```python
from build123d import *

# Parameters (mm, degrees)
SKETCH1_R           = 2
SKETCH1_R_2         = 1.5
BOSS_EXTRUDE1_DEPTH = 1.5
SCALE1_SCALE        = 1.5
FILLET1_R           = 0.75


with BuildPart() as part:
    # Sketch1 → Boss-Extrude1 (new, symmetric)
    with BuildSketch(Plane(origin=(0, 0, 0), x_dir=(1, 0, 0), z_dir=(0, 1, 0))):
        with BuildLine():
            ThreePointArc((-18.5, 4), (-22.5, 0), (-18.5, -4))
            Line((-18.5, -4), (-12.5, -4))
            ThreePointArc((-12.5, -4), (-10.036924503, -2.516685226), (-7.208497378, -2))
            Line((-7.208497378, -2), (8.627016654, -2))
            ThreePointArc((8.627016654, -2), (10.627016654, -2.254033308), (12.5, -3))
            Line((12.5, -3), (18.5, -3))
            ThreePointArc((18.5, -3), (21.5, 0), (18.5, 3))
            Line((18.5, 3), (12.5, 3))
            ThreePointArc((12.5, 3), (10.627016654, 2.254033308), (8.627016654, 2))
            Line((8.627016654, 2), (-7.208497378, 2))
            ThreePointArc((-7.208497378, 2), (-10.036924503, 2.516685226), (-12.5, 4))
            Line((-12.5, 4), (-18.5, 4))
        make_face()
        with Locations(Location((-18.5, 0, 0), (0, 0, 270))):
            Circle(SKETCH1_R, mode=Mode.SUBTRACT)
        with Locations(Location((18.5, 0, 0), (0, 0, 270))):
            Circle(SKETCH1_R_2, mode=Mode.SUBTRACT)
    extrude(amount=BOSS_EXTRUDE1_DEPTH, both=True)


with BuildPart() as part_1:
    # Scale1: scaled about (-1.682409561, 0, 0)
    add(part.part.scale(SCALE1_SCALE).moved(Location((0.841204781, 0, 0))))

    # Fillet1
    fillet1_edges = [part_1.edges().sort_by_distance(p)[0] for p in [
        (33.09120478, 2.25, 0),
        (24.091204781, 2.25, -4.5),
        (16.781729761, -2.25, 3.381049961),
        (1.905094237, -2.25, 3),
        (-14.214181973, -2.25, 3.77502784),
        (-22.408795219, -2.25, 6),
        (-32.908795219, -2.25, 0),
        (-22.408795219, -2.25, -6),
        (-14.214181973, -2.25, -3.77502784),
        (1.905094237, -2.25, -3),
        (16.781729761, -2.25, -3.381049961),
        (24.091204781, -2.25, -4.5),
        (16.781729761, 2.25, -3.381049961),
        (33.09120478, -2.25, 0),
        (24.091204781, -2.25, 4.5),
        (1.905094237, 2.25, -3),
        (-14.214181973, 2.25, -3.77502784),
        (-22.408795219, 2.25, -6),
        (-32.908795219, 2.25, 0),
        (-22.408795219, 2.25, 6),
        (-14.214181973, 2.25, 3.77502784),
        (1.905094237, 2.25, 3),
        (16.781729761, 2.25, 3.381049961),
        (24.091204781, 2.25, 4.5),
    ]]
    fillet(fillet1_edges, radius=FILLET1_R)


solid = part_1.part
```
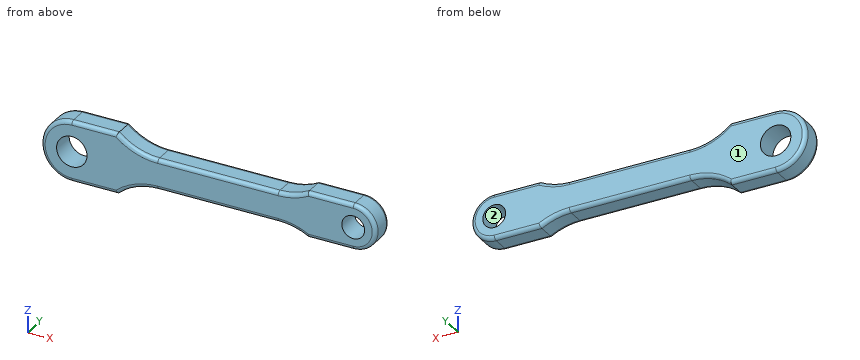
Can you work these out from the model? Positions are in its coordinate system, mm. Face numbers are marked on the shaded views. Give positions to 0.01 mm unless a question says otherwise; leave off trailing zeros. Loops run counter-clockwise (first coordinate to the right, second up) from the corner with the lowest first, then second, coordinate; pieces in that order, holes last. Notation, with made-up numbers: M -15.5,22.5 L 19.5,22.5 A22 cw 19.5,54.5 Z; hole C -1,0 d1. An arc over 180 degrees is marked long. One line per item, written item: value.
(1) Suppose I cut it at B-B on y = 0.95. List the corners of the cut face in (x, z) for me.
Returned:
outline: M -26.91,-6 L -17.91,-6 A12 cw -9.97,-3 L 13.78,-3 A12 cw 19.59,-4.5 L 28.59,-4.5 A4.5 ccw 28.59,4.5 L 19.59,4.5 A12 cw 13.78,3 L -9.97,3 A12 cw -17.91,6 L -26.91,6 A6 ccw Z; hole C -26.91,0 d6; hole C 28.59,0 d4.5
(2) I need wall thicknesses on line 1 (X direction, y = 0.95, z = 0); line 2 (X direction, y = 2.05, z = -2); line 3 (Z direction, x = -7, y = 1.35). Which ranges of each line are inside material? Lowest first, please.
Returned:
line 1: -32.91 to -29.91, -23.91 to 26.34, 30.84 to 33.09
line 2: -32.31 to -29.14, -24.67 to 27.56, 29.62 to 32.35
line 3: -3 to 3
(3) Will these pins go through, and if not, where does the flat tip stop? pin 1 (2.5 mm diameter, centred on x = 3, y = -0.5, fed in from -Z); pin 2 (2.5 mm diameter, centred on x = 22.5, y = 0.5, fed in from +Z); pin 3 (2.5 mm diameter, centred on x = 24, y = 0, fed in from -Z).
Returned:
pin 1: z = -3
pin 2: z = 4.5
pin 3: z = -4.5
(4) Suppose I cut it at C-C on x = 24.5. List the corners of the cut face in (y, z) for me.
Returned:
outline: M -2.25,-3.75 A0.75 ccw -1.5,-4.5 L 1.5,-4.5 A0.75 ccw 2.25,-3.75 L 2.25,3.75 A0.75 ccw 1.5,4.5 L -1.5,4.5 A0.75 ccw -2.25,3.75 Z
(5) We'd pull the mould along X, two halves only. Please class the marked faces 1 and 2: released by +X, released by -X, zero draft, split by the parting line, or undercut.
Returned:
face 1: zero draft
face 2: undercut
(6) Suppose I cut it at A-A on z = 0. List the corners of the cut face in (x, y) for me, plus the area to 3 significant figures.
Returned:
outline: M -32.91,-1.5 A0.75 ccw -32.16,-2.25 L -29.91,-2.25 L -29.91,2.25 L -32.16,2.25 A0.75 ccw -32.91,1.5 Z; M -23.91,-2.25 L 26.34,-2.25 L 26.34,2.25 L -23.91,2.25 Z; M 30.84,-2.25 L 32.34,-2.25 A0.75 ccw 33.09,-1.5 L 33.09,1.5 A0.75 ccw 32.34,2.25 L 30.84,2.25 Z
area: 249 mm^2
(7) Suppose I cut it at D-D on x = -25. List the corners of the cut face in (y, z) for me, plus the area to 3 significant figures.
Returned:
outline: M -2.25,-5.25 A0.75 ccw -1.5,-6 L 1.5,-6 A0.75 ccw 2.25,-5.25 L 2.25,-2.31 L -2.25,-2.31 Z; M -2.25,2.31 L 2.25,2.31 L 2.25,5.25 A0.75 ccw 1.5,6 L -1.5,6 A0.75 ccw -2.25,5.25 Z
area: 32.7 mm^2
